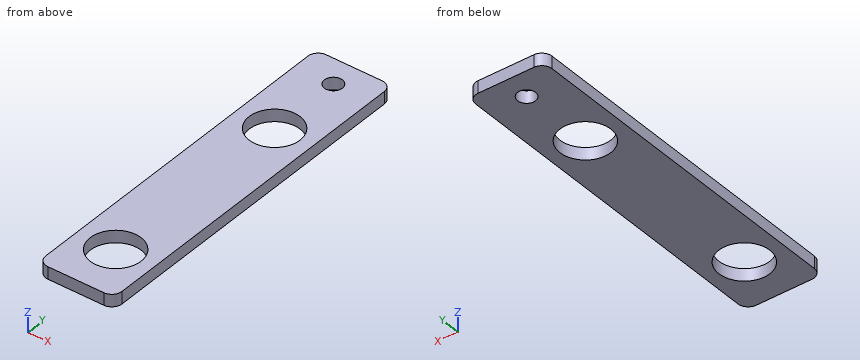
from build123d import *

# Parameters (mm, degrees)
SKETCH1_W             = 19.05
SKETCH1_H             = 88.9
SKETCH1_R             = 6.35
BOSS_EXTRUDE1_DEPTH   = 3.0734
F_8_CLEARANCE_HOLE1_D = 4.4958
FILLET1_R             = 2.54


with BuildPart() as part:
    # Sketch1 → Boss-Extrude1 (new body)
    with BuildSketch(Plane.XY):
        with Locations((9.525, 44.45)):
            Rectangle(SKETCH1_W, SKETCH1_H)
        with Locations((9.525, 12.7)):
            Circle(SKETCH1_R, mode=Mode.SUBTRACT)
        with Locations((9.525, 63.5)):
            Circle(SKETCH1_R, mode=Mode.SUBTRACT)
    extrude(amount=BOSS_EXTRUDE1_DEPTH)

    # #8 Clearance Hole1 (through all)
    with Locations(Plane.XY.offset(3.0734)):
        with Locations((9.627458059, 82.1563)):
            Hole(F_8_CLEARANCE_HOLE1_D / 2)

    # Fillet1
    fillet1_edges = [part.edges().sort_by_distance(p)[0] for p in [
        (0, 88.9, 1.5367),
        (19.05, 88.9, 1.5367),
        (19.05, 0, 1.5367),
        (0, 0, 1.5367),
    ]]
    fillet(fillet1_edges, radius=FILLET1_R)


solid = part.part
Build history of the part. All positions in model axes, mm. Coordinates: 2 decimals unless noted, no trailing zeros. Order: outer loops, then holes, each group sorted by start corner. A loop starts at its lowest first (then second) coordinate and runs counter-clockwise, first axis right, second up. Notation, with made-up numbers: (58, 88) - (101, 88) arc R21 ccw to (101, 109) - close; hole circle Ø8 at (9, 70.5). An arc over 180 degrees is marked (long way). Write each question's results on one line, items separated by ' | '. Start each with the question number.
Item 1: Band-saw the part on A-A on y = 63.5. Write the cut outline in (x, z) (3 decimals).
Item 2: Wall check: probe 1 along Y at (x, z) = (9.5, 0.4); probe 2 along Y at (x, z) = (13.75, 1.15); probe 3 along Y at (x, z) = (6, 2.4). Give the ranges that are in metal, low to high. Write a range as [from, to].
Item 3: Band-saw the part on C-C on z = 2.35. Write the cut outline in (x, y) (3 decimals), and give its area (3 significant figures).
Item 4: Band-saw the part on B-B on x = 8.5. Write the cut outline in (y, z), and give its area (3 significant figures).
Numbers:
1) outline: (0, 0) - (3.175, 0) - (3.175, 3.073) - (0, 3.073) - close; (15.875, 0) - (19.05, 0) - (19.05, 3.073) - (15.875, 3.073) - close
2) probe 1: [0, 6.35], [19.05, 57.15], [69.85, 79.91], [84.4, 88.9] | probe 2: [0, 7.96], [17.44, 58.76], [68.24, 88.9] | probe 3: [0, 7.42], [17.98, 58.22], [68.78, 88.9]
3) outline: (0, 2.54) arc R2.54 ccw to (2.54, 0) - (16.51, 0) arc R2.54 ccw to (19.05, 2.54) - (19.05, 86.36) arc R2.54 ccw to (16.51, 88.9) - (2.54, 88.9) arc R2.54 ccw to (0, 86.36) - close; hole circle Ø12.7 at (9.525, 12.7); hole circle Ø12.7 at (9.525, 63.5); hole circle Ø4.496 at (9.627, 82.156) | area: 1,420 mm^2
4) outline: (0, 0) - (6.43, 0) - (6.43, 3.07) - (0, 3.07) - close; (18.97, 0) - (57.23, 0) - (57.23, 3.07) - (18.97, 3.07) - close; (69.77, 0) - (80.21, 0) - (80.21, 3.07) - (69.77, 3.07) - close; (84.1, 0) - (88.9, 0) - (88.9, 3.07) - (84.1, 3.07) - close | area: 184 mm^2
